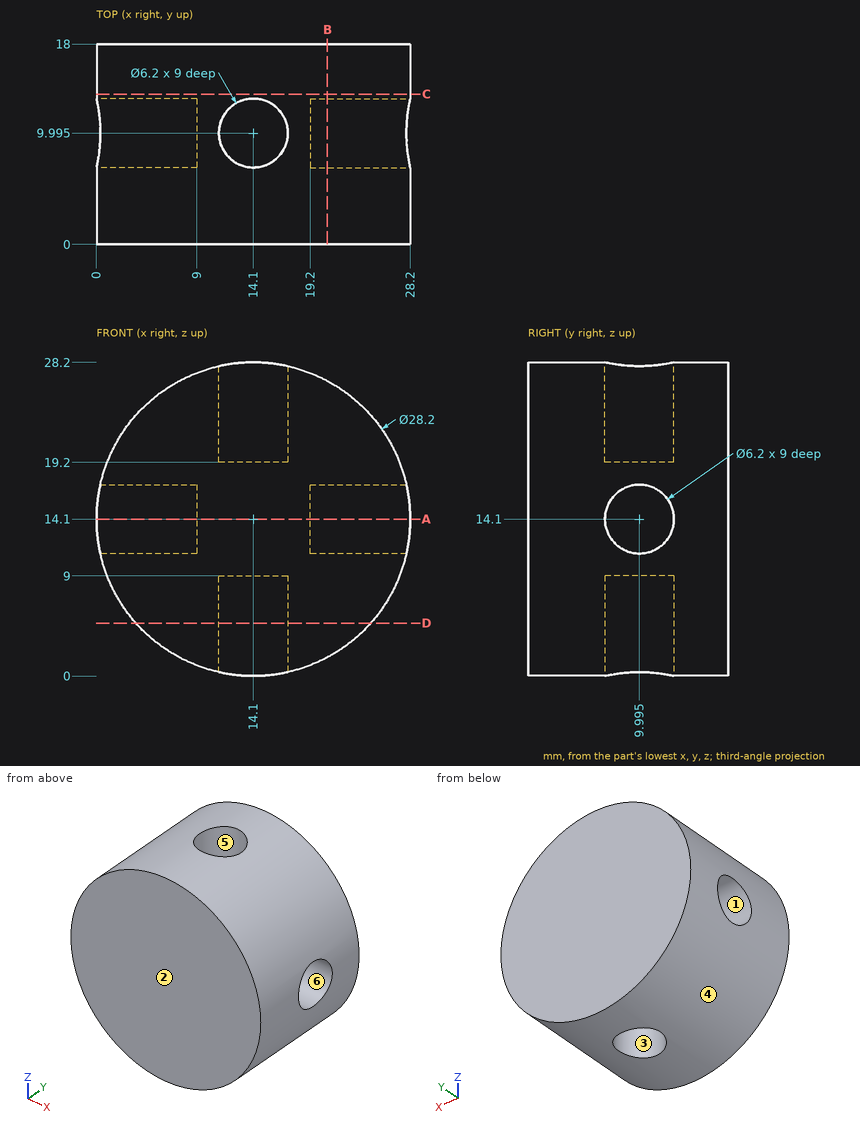
Design review of the part shown in the three views and the two pictorial views. Dimensions are in mm from the part's minimum x, y and z. A direction names the side the tool comes from. Round coordinates to 2 decimals unless told otherwise and drop trailing zeros. Write each loop counter-clockwise with the first axis right and the second up, starting at its lowest first coordinate (ties: lowest second). Pieces come first, ordered by that corner, then holes. Notation, with made-up numbers: (45.5, 54.25) - (66.5, 54.25) arc R5 cw to (66.5, 61.25) - close; hole circle Ø2 at (-0.5, -17.75). An arc over 180 degrees is marked (long way). Write item = value, one per line. Start each with the question number.
1. For pin 1 Ø1.5 at (x, y) = (16, 5) entering from -Z; pin 2 Ø5 at (y, z) = (10, 14.1) entering from +X; pin 3 Ø5.5 at (x, y) = (14.1, 10) entering from +Z, all flat-tipped, find the tip position at first contact; note any pin that passes through.
2. Draft analysis for pull direction Z (two halves, no side actions). For the marked faces 4, 5 and 6, state which applies: released by +Z, released by -Z, zero draft, split by the parting line, or undercut.
3. Consider section D-D on z = 4.75. State the section outline as (x, y) points (1 decimal), plus the area to 3 significant figures.
4. Consider section C-C on y = 13.5. State the section outline as (x, z) points.
5. Consider section A-A on z = 14.1. State the section outline as (x, y) points (1 decimal), plus the area to 3 significant figures.
6. Wall thickness on L1, parallel to Y at x = 14.25, z = 24; L2, parallel to X at y = 11.5, z = 3 (1 decimal); L3, parallel to Z at x = 17, y = 10.5: over which ranges is each line inside the solid? List them lowest first.
7. For the marked faces 1, 2 and 3, list the 3-axis set-ups (+Z, -Z, +X, -X, +Y, -Y) from which the entire face can be reached by the end or side of a thin tool; tool diameter is ignored.
8. Consider section B-B on x = 20.75. State the section outline as (y, z) points (1 decimal).
Evaluation:
q1.pin_1 = 0.05
q1.pin_2 = 19.2
q1.pin_3 = 19.2
q2.face_4 = split by the parting line
q2.face_5 = zero draft
q2.face_6 = undercut
q3.outline = (3.5, 0) - (24.7, 0) - (24.7, 18) - (3.5, 18) - close; hole circle Ø6.2 at (14.1, 10)
q3.area = 350 mm2
q4.outline = circle Ø28.2 at (14.1, 14.1)
q5.outline = (0, 0) - (28.2, 0) - (28.2, 6.9) - (19.2, 6.9) - (19.2, 13.1) - (28.2, 13.1) - (28.2, 18) - (0, 18) - (0, 13.1) - (9, 13.1) - (9, 6.9) - (0, 6.9) - close
q5.area = 396 mm2
q6.L1 = 0 to 6.9, 13.09 to 18
q6.L2 = 5.4 to 11.4, 16.8 to 22.8
q6.L3 = 9 to 19.2
q7.face_1 = -X
q7.face_2 = +Z, -Z, +X, -X, -Y
q7.face_3 = -Z
q8.outline = (0, 1.7) - (18, 1.7) - (18, 26.5) - (0, 26.5) - close; hole circle Ø6.2 at (10, 14.1)
